Build history of the part. All positions in model axes, mm. Face numbers are marked on the shaded views. A direction names the side the tool comes from. Coordinates: 2 decimals unless noted, no trailing zeros. Order: outer loops, then holes, each group sorted by start corner. A loop starts at its lowest first (then second) coordinate and runs counter-clockwise, first axis right, second up. Notation, with made-up numbers: (23, 54.5) - (73, 54.5) arc R24 cw to (73, 79.5) - close; hole circle Ø5 at (49, 89). An arc over 180 degrees is marked (long way). Write each question's results on one line, items separated by ' | '. Start each with the question number.
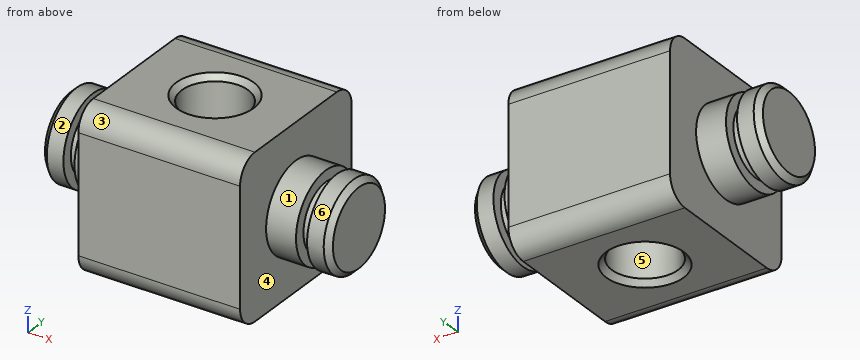
from build123d import *

# Parameters (mm, degrees)
SKETCH1_W                = 14.6
SKETCH1_H                = 14.6
BOSS_EXTRUDE1_DEPTH      = 15
SKETCH2_R                = 3
CUT_EXTRUDE1_DEPTH       = 14.6
CHAMFER1_SIZE            = 0.5
SKETCH3_R                = 4
BOSS_EXTRUDE2_DEPTH      = 5.7
SKETCH4_W                = 1
SKETCH4_H                = 1.778268535
CHAMFER2_SIZE            = 0.5
CHAMFER2_OF_MIRROR1_SIZE = 0.5
FILLET1_R                = 2


with BuildPart() as part:
    # Sketch1 → Boss-Extrude1 (new body)
    with BuildSketch(Plane(origin=(0, 0, 0), x_dir=(1, 0, 0), z_dir=(0, 1, 0))):
        Rectangle(SKETCH1_W, SKETCH1_H)
    extrude(amount=BOSS_EXTRUDE1_DEPTH)

    # Sketch2 → Cut-Extrude1 (cut)
    with BuildSketch(Plane(origin=(0, 7.7, -7.3), x_dir=(1, 0, 0), z_dir=(0, 0, 1))):
        with Locations((0, -0.2)):
            Circle(SKETCH2_R)
    extrude(amount=CUT_EXTRUDE1_DEPTH, mode=Mode.SUBTRACT)

    # Chamfer1
    chamfer1_edges = [part.edges().sort_by_distance(p)[0] for p in [
        (-3, 7.5, -7.3),
        (-3, 7.5, 7.3),
    ]]
    chamfer(chamfer1_edges, length=CHAMFER1_SIZE)

    # Sketch3 → Boss-Extrude2 (add)
    with BuildSketch(Plane.ZY.offset(7.3)):
        with Locations((0, 7.5)):
            Circle(SKETCH3_R)
    boss_extrude2 = extrude(amount=BOSS_EXTRUDE2_DEPTH)

    # Sketch4 → Cut-Revolve1 (revolve, cut)
    with BuildSketch(Plane.XY):
        with Locations((-10.5, 11.389134268)):
            Rectangle(SKETCH4_W, SKETCH4_H)
    cut_revolve1 = revolve(axis=Axis((-13, 7.5, 0), (1, 0, 0)), mode=Mode.SUBTRACT)

    # Chamfer2
    chamfer2_edges = [part.edges().sort_by_distance(p)[0] for p in [
        (-13, 7.5, -4),
    ]]
    chamfer(chamfer2_edges, length=CHAMFER2_SIZE)

    # Mirror1: Boss-Extrude2, Cut-Revolve1 across plane
    add(boss_extrude2.mirror(Plane(origin=(0, 0, 0), x_dir=(0, 0, 1), z_dir=(1, 0, 0))))
    add(cut_revolve1.mirror(Plane(origin=(0, 0, 0), x_dir=(0, 0, 1), z_dir=(1, 0, 0))), mode=Mode.SUBTRACT)

    # Chamfer2 of Mirror1
    chamfer2_of_mirror1_edges = [part.edges().sort_by_distance(p)[0] for p in [
        (13, 7.5, -4),
    ]]
    chamfer(chamfer2_of_mirror1_edges, length=CHAMFER2_OF_MIRROR1_SIZE)

    # Fillet1
    fillet1_edges = [part.edges().sort_by_distance(p)[0] for p in [
        (0, 15, -7.3),
        (0, 0, -7.3),
        (0, 0, 7.3),
        (0, 15, 7.3),
    ]]
    fillet(fillet1_edges, radius=FILLET1_R)


solid = part.part
Item 1: Slice it at C-C (x = 5.25). Write the cut outline in (y, z).
Item 2: Pull direction Y, two halves, no side cores. Call the marked faces 4, 5 and 6: released by +Y, released by -Y, zero draft, split by the parting line, or undercut.
Item 3: Slice it at A-A (x = 0). Write the cut outline in (y, z).
Item 4: Flat gauge pin, fed straight in: P1, Ø1, axis at x = -8.5, y = 6.5, coming from the +Z side. Where does the tip first touch, or does it go through?
Item 5: Slice it at D-D (z = 6). Write the cut outline in (x, y).
Item 6: Probe probe 1 along Y at (x, z) = (0, -2); probe 2 along X at (y, z) = (7, -3.75); probe 3 along X at (y, z) = (4.75, 5). List the from-to ranges inside material, lowest first.
Item 7: Which spindle directions (+Z, -Z, +X, -X, +Y, -Y) get a long thin tool onto all of the face, cutting with end or side? Do the marked faces 1, 2 and 3. Say none if no direction does.
Resolved:
1) outline: (0, -5.3) arc R2 ccw to (2, -7.3) - (13, -7.3) arc R2 ccw to (15, -5.3) - (15, 5.3) arc R2 ccw to (13, 7.3) - (2, 7.3) arc R2 ccw to (0, 5.3) - close
2) face 4: zero draft | face 5: undercut | face 6: split by the parting line
3) outline: (0, -5.3) arc R2 ccw to (2, -7.3) - (4, -7.3) - (4.5, -6.8) - (4.5, 6.8) - (4, 7.3) - (2, 7.3) arc R2 ccw to (0, 5.3) - close; (10.5, -6.8) - (11, -7.3) - (13, -7.3) arc R2 ccw to (15, -5.3) - (15, 5.3) arc R2 ccw to (13, 7.3) - (11, 7.3) - (10.5, 6.8) - close
4) P1: z = 3.97
5) outline: (-7.3, 0.13) - (7.3, 0.13) - (7.3, 14.87) - (-7.3, 14.87) - close; hole circle Ø6 at (0, 7.5)
6) probe 1: 0 to 4.5, 10.5 to 15 | probe 2: -12.72 to -11, -10 to -2.96, 2.96 to 10, 11 to 12.72 | probe 3: -7.3 to -1.2, 1.2 to 7.3
7) face 1: +X | face 2: -X | face 3: +Z, +X, -X, -Y
